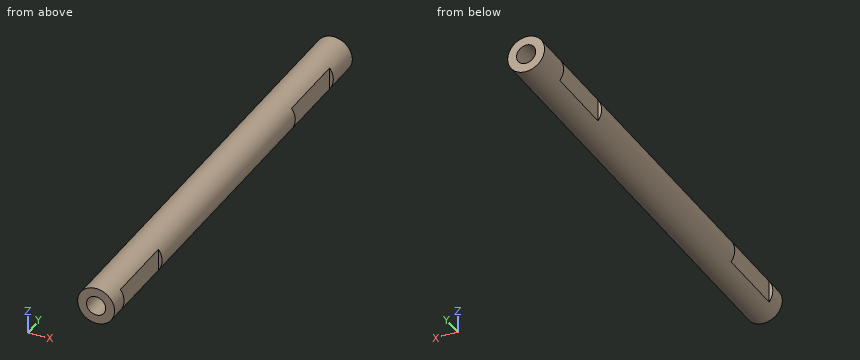
```python
from build123d import *

# Parameters (mm, degrees)
SKETCH_1_R          = 5
EXTRUDE_1_DEPTH     = 125
M5X0_8_D            = 5.2
M5X0_8_DEPTH        = 16
M5X0_8_TIP          = 1.562237609
M5X0_8_2_D          = 5.2
M5X0_8_2_DEPTH      = 16
M5X0_8_2_TIP        = 1.562237609
CUT_EXTRUDE_START   = -20
CUT_EXTRUDE_5_DEPTH = 20
CUT_EXTRUDE_6_DEPTH = 20


with BuildPart() as part:
    # ｽｹｯﾁ1 → ﾎﾞｽ - 押し出し1 (new body)
    with BuildSketch(Plane(origin=(0, 0, 0), x_dir=(1, 0, 0), z_dir=(0, 1, 0))):
        with Locations(Location((0, 0, 0), (0, 0, 270))):
            Circle(SKETCH_1_R)
    extrude(amount=EXTRUDE_1_DEPTH)

    # M5x0.8
    with Locations(Plane.ZX.offset(125)):
        with Locations((0, 0)):
            Hole(M5X0_8_D / 2, depth=M5X0_8_DEPTH)
            with Locations((0, 0, -(M5X0_8_DEPTH + M5X0_8_TIP / 2))):  # 118° drill point
                Cone(0, M5X0_8_D / 2, M5X0_8_TIP, mode=Mode.SUBTRACT)

    # M5x0.8 2
    with Locations(Plane(origin=(0, 0, 0), x_dir=(0, 0, -1), z_dir=(0, -1, 0))):
        with Locations((0, 0)):
            Hole(M5X0_8_2_D / 2, depth=M5X0_8_2_DEPTH)
            with Locations((0, 0, -(M5X0_8_2_DEPTH + M5X0_8_2_TIP / 2))):  # 118° drill point
                Cone(0, M5X0_8_2_D / 2, M5X0_8_2_TIP, mode=Mode.SUBTRACT)

    # ｽｹｯﾁ8 → ｶｯﾄ - 押し出し5 (cut)
    with BuildSketch(Plane(origin=(0, 115, 0), x_dir=(1, 0, 0), z_dir=(0, 1, 0)).offset(CUT_EXTRUDE_START)):
        with BuildLine():
            ThreePointArc((4, 3), (5, 0), (4, -3))
            Line((4, -3), (4, 3))
        make_face()
        with BuildLine():
            Line((-4, -2.309397765), (-4, 0))
            Line((-4, 0), (-5, 0))
            ThreePointArc((-5, 0), (-4.74341649, -1.58113883), (-4, -3))
            Line((-4, -3), (-4, -2.309397765))
        make_face()
        with BuildLine():
            Line((-5, 0), (-4, 0))
            Line((-4, 0), (-4, 3))
            ThreePointArc((-4, 3), (-4.74341649, 1.58113883), (-5, 0))
        make_face()
    extrude(amount=CUT_EXTRUDE_5_DEPTH, mode=Mode.SUBTRACT)

    # ｽｹｯﾁ9 → ｶｯﾄ - 押し出し6 (cut)
    with BuildSketch(Plane(origin=(0, 5, 0), x_dir=(-1, 0, 0), z_dir=(0, -1, 0))):
        with BuildLine():
            Line((-4, 3), (-4, -3))
            ThreePointArc((-4, -3), (-5, 0), (-4, 3))
        make_face()
        with BuildLine():
            Line((4, -3), (4, 3))
            ThreePointArc((4, 3), (5, 0), (4, -3))
        make_face()
    extrude(amount=-CUT_EXTRUDE_6_DEPTH, mode=Mode.SUBTRACT)


solid = part.part
```
Read the model definition and answer for the solid it produces. Units are mm, in the model's axes. Round coordinates to 2 decimals unless told otherwise and drop trailing zeros. Write each loop counter-clockwise with the first axis right and the second up, starting at its lowest first coordinate (ties: lowest second). Pieces come first, ordered by that corner, then holes. Notation, with made-up numbers: M -19.5,-16.5 L 11.5,-16.5 A14 ccw 11.5,5.5 Z; hole C 48.5,10 d7. An arc over 180 degrees is marked long. One line per item, written item: value.
Q1. Find section B-B on y = 84. Write down the section's boundary in (x, z).
Data:
outline: C 0,0 d10
Q2. Find section A-A on y = 14. Write down the section's boundary in (x, z), plus the area to 3 significant figures.
Data:
outline: M -4,-3 A5 ccw 4,-3 L 4,3 A5 ccw -4,3 Z; hole C 0,0 d5.2
area: 49.1 mm2
Q3. Straight lines are drawn through the part: line 1 (Y direction, x = 4.25, z = -0.75); line 2 (X direction, y = 118.75, z = 0); line 3 (Z direction, x = -4, y = 30). For each, find the intervals that lie inside material, in ascending order. Write a range as [from, to].
Data:
line 1: [0, 5], [25, 95], [115, 125]
line 2: [-5, -2.6], [2.6, 5]
line 3: [-3, 3]
Q4. Flat-ended cylindrical pins translate along their axes: pin 1 Ø5 at (y, z) = (102, -0.5) entering from +X; pin 2 Ø2 at (y, z) = (35, -1.5) entering from -X; pin 3 Ø4 at (x, z) = (0, 0) entering from +Y. Find the tip coordinate at first contact, or state that the pin passes through.
Data:
pin 1: x = 4
pin 2: x = -4.97
pin 3: y = 108.64
